Autodesk Inventor part; units mm, degrees
ref_plane "to_screw_XY" through (0, 0, 0) normal (0, -1, 0) x (1, 0, 0)
ref_plane "to_screw_YZ" through (0, 0, 0) normal (1, 0, 0) x (0, 0, 1)
ref_plane "to_screw_ZX" through (0, 0, 0) normal (0, 0, 1) x (0, -1, 0)
sketch "Sketch_1" plane through (0, 0, 0) normal (0, 0, 1) x (1, 0, 0)
  line L0 (-12.7, 4.064) -> (-12.7, 0)
  line L1 (-12.7, 0) -> (12.7, 0)
  line L2 (12.7, 0) -> (12.7, 4.064)
  line L3 (12.7, 4.064) -> (3.556, 4.064)
  arc A0 (2.921, 4.699) -> (3.556, 4.064) centre (3.556, 4.699) ccw
  line L4 (2.921, 4.699) -> (2.921, 6.223)
  arc A1 (3.556, 6.858) -> (2.921, 6.223) centre (3.556, 6.223) ccw
  line L5 (3.556, 6.858) -> (6.3764, 6.858)
  line L6 (6.3764, 6.858) -> (6.3764, 7.366)
  line L7 (6.3764, 7.366) -> (2.54, 11.938)
  line L8 (2.54, 11.938) -> (-2.54, 11.938)
  line L9 (-2.54, 11.938) -> (-6.3764, 7.366)
  line L10 (-6.3764, 7.366) -> (-6.3764, 6.858)
  line L11 (-6.3764, 6.858) -> (-3.556, 6.858)
  arc A2 (-2.921, 6.223) -> (-3.556, 6.858) centre (-3.556, 6.223) ccw
  line L12 (-2.921, 6.223) -> (-2.921, 4.699)
  arc A3 (-3.556, 4.064) -> (-2.921, 4.699) centre (-3.556, 4.699) ccw
  line L13 (-3.556, 4.064) -> (-12.7, 4.064)
extrude "Extrusion1" add sketch "Sketch_1" along normal mid plane 25.4
sketch "Sketch_2" plane through (0, 11.938, 0) normal (0, 1, 0) x (1, 0, 0)
  line L0 (-2.3749, 6.604) -> (-2.3749, -6.604)
  arc A0 (-2.3749, -6.604) -> (2.3749, -6.604) centre (0, -6.604) ccw
  line L1 (2.3749, -6.604) -> (2.3749, 6.604)
  arc A1 (2.3749, 6.604) -> (-2.3749, 6.604) centre (0, 6.604) ccw
extrude "Extrusion2" cut sketch "Sketch_2" against normal blind 4.318
sketch "Sketch3" plane through (-12.7, 0, 12.7) normal (0, -1, 0) x (1, 0, 0)
  point P0 (12.7, -12.7)
hole "Hole1" at (0, 0, 0) direction (0, 1, 0) diameter 6.5278 depth 11.938
ref_plane "to_screw_XY" through (0, 0, 0) normal (0, -1, 0) x (1, 0, 0)
ref_plane "to_screw_YZ" through (0, 0, 0) normal (1, 0, 0) x (0, 0, 1)
ref_plane "to_screw_ZX" through (0, 0, 0) normal (0, 0, 1) x (0, -1, 0)
properties part number "2059_a"
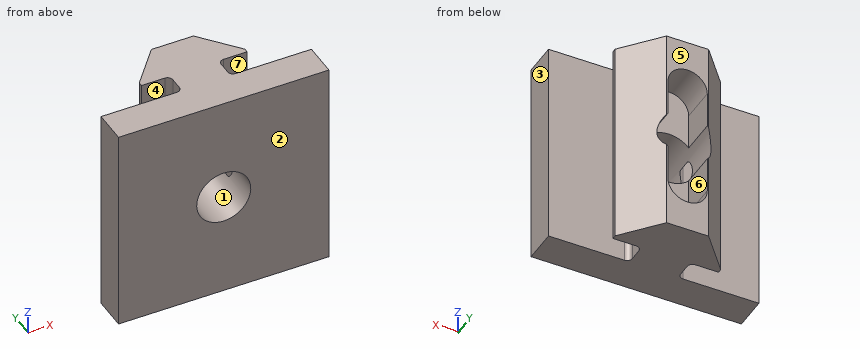
Here's how the part is built. I have some questions about the finished solid (model axes, mm). Face numbers are marked on the shaded views. A direction names the side the tool comes from. Give positions to 0.01 mm unless a question says otherwise; leave off trailing zeros. Loops run counter-clockwise (first coordinate to the right, second up) from the corner with the lowest first, then second, coordinate; pieces in that order, holes last. Notation, with made-up numbers: (78, 25) -> (86, 25) arc R19 cw to (86, 51) -> close; hole circle Ø10 at (89.25, -19). An arc over 180 degrees is marked (long way). Use one line per item in the form item = value. Start each with the question number.
1) Please list where these lines run through material, in increasing order: line 1 along X through (y, z) = (4, 0); line 2 along Z through (x, y) = (0, 9); line 3 along Y through (x, z) = (-11, 8.5).
2) For P1, Ø1.7, axis at y = 5.5, z = -5, coming from the -X side; P2, Ø2.5, axis at x = -9, z = 3, coming from the +Y side; P3, Ø0.5, axis at y = 5, z = 7.5, coming from the +X side, each with a flat end and sliding along its axis, tell me the tip position at first contact or that it passes through.
3) Imagine slicing it at C-C (z = -4.75). Please give me the cut outline in (x, y) (3 decimals).
4) Imagine slicing it at A-A (x = 0). Please give me the cut outline in (y, z), then the cut area to 3 significant figures.
5) Imagine slicing it at B-B (z = 0). Please give me the cut outline in (x, y) (3 decimals).
6) Thinking about a two-plate mould opening in X: for the marked faces 1, 2 and 3, which applies, +X half, -X half, draft (parallel to the pull), parting line (faces both ways), or undercut?
7) Imagine slicing it at D-D (y = 3.5). Please give me the cut outline in (x, z), then the cut area to 3 significant figures.
8) Which directions (+Z, -Z, +X, -X, +Y, -Y) give clear straight access to the entire face, cutting with the end or side of a thin tool? Please do the marked faces 4, 5, 6 and 7.
Check values:
q1.line_1 = -12.7 to -3.26, 3.26 to 12.7
q1.line_2 = -12.7 to -8.98, 8.98 to 12.7
q1.line_3 = 0 to 4.06
q2.P1 = -2.93
q2.P2 = 4.06
q2.P3 = 2.92
q3.outline = (-12.7, 0) -> (12.7, 0) -> (12.7, 4.064) -> (3.556, 4.064) arc R0.635 cw to (2.921, 4.699) -> (2.921, 6.223) arc R0.635 cw to (3.556, 6.858) -> (6.376, 6.858) -> (6.376, 7.366) -> (2.54, 11.938) -> (2.375, 11.938) -> (2.375, 7.62) -> (-2.375, 7.62) -> (-2.375, 11.938) -> (-2.54, 11.938) -> (-6.376, 7.366) -> (-6.376, 6.858) -> (-3.556, 6.858) arc R0.635 cw to (-2.921, 6.223) -> (-2.921, 4.699) arc R0.635 cw to (-3.556, 4.064) -> (-12.7, 4.064) -> close
q4.outline = (0, -12.7) -> (11.94, -12.7) -> (11.94, -8.98) -> (7.62, -8.98) -> (7.62, -3.26) -> (0, -3.26) -> close; (0, 3.26) -> (7.62, 3.26) -> (7.62, 8.98) -> (11.94, 8.98) -> (11.94, 12.7) -> (0, 12.7) -> close
q4.area = 176 mm^2
q5.outline = (-12.7, 0) -> (-3.264, 0) -> (-3.264, 4.135) arc R0.635 cw to (-3.556, 4.064) -> (-12.7, 4.064) -> close; (-6.376, 6.858) -> (-3.556, 6.858) arc R0.635 cw to (-3.264, 6.787) -> (-3.264, 11.075) -> (-6.376, 7.366) -> close; (3.264, 0) -> (12.7, 0) -> (12.7, 4.064) -> (3.556, 4.064) arc R0.635 cw to (3.264, 4.135) -> close; (3.264, 6.787) arc R0.635 cw to (3.556, 6.858) -> (6.376, 6.858) -> (6.376, 7.366) -> (3.264, 11.075) -> close
q6.face_1 = undercut
q6.face_2 = draft
q6.face_3 = +X half
q7.outline = (-12.7, -12.7) -> (12.7, -12.7) -> (12.7, 12.7) -> (-12.7, 12.7) -> close; hole circle Ø6.53 at (0, 0)
q7.area = 612 mm^2
q8.face_4 = +Z, -Z, -X
q8.face_5 = +Z, -Z, +X, -X, +Y
q8.face_6 = +Y
q8.face_7 = +Z, -Z, +X
